Verification items for the finished model (mm, model axes). A direction names the side the tool comes from. Give positions to 0.01 mm unless a question says otherwise; leave off trailing zeros. Loops run counter-clockwise (first coordinate to the right, second up) from the corner with the lowest first, then second, coordinate; pieces in that order, holes last. Notation, with made-up numbers: (47.5, 35) - (98.5, 35) arc R28 ccw to (98.5, 60) - close; hole circle Ø8 at (-2, -37.75). An arc over 180 degrees is marked (long way). Answer in a Markdown table with one row per item.
```python
from build123d import *

# Parameters (mm, degrees)
F1_DEPTH = 254


with BuildPart() as f1:
    # F0 (on Front) → F1 (new body)
    with BuildSketch(Plane.XZ):
        Polygon((124.411419, 0), (0, 0), (0, -63.5), (63.5, -63.5), (48.04277, -25.4), (201.770738, -25.4), (190.5, -63.5), (254, -63.5), (254, 0), align=None)
        with BuildLine():
            Line((37.633552, 108.208333), (0, 0))
            Line((0, 0), (124.411419, 0))
            ThreePointArc((124.411419, 0), (55.058262, 33.282111), (37.633552, 108.208333))
        make_face()
        with BuildLine():
            ThreePointArc((213.311419, 88.9), (187.273212, 26.038207), (124.411419, 0))
            Line((124.411419, 0), (254, 0))
            Line((254, 0), (211.189286, 108.208333))
            ThreePointArc((211.189286, 108.208333), (212.779293, 98.612301), (213.311419, 88.9))
        make_face()
    extrude(amount=F1_DEPTH)


solid = f1.part
```
Q1. Draft check along Z on faces 1 (the face through (212.764, -125.222, 98.748)), 2 (the face through (0, -125, -31)), 3 (the face through (222, -125, -63.5)). Enter one of: +Z half, -Z half, draft (parallel to the pull), parting line (faces both ways), or undercut.
Completed:
| item | result |
|---|---|
| face 1 | undercut |
| face 2 | draft |
| face 3 | -Z half |
Q2. Go/stop test with flat-tipped pins: P1, Ø3, axis at x = 86.5, y = -25.5, coming from the +Z side; P2, Ø1.5, axis at y = -225, z = 46, coming from the -X side; P3, Ø3, axis at x = 171.5, y = -197.5, coming from the -Z side. Record where each tip stops, or that it passes through.
Completed:
| item | result |
|---|---|
| P1 | z = 9.21 |
| P2 | x = 15.74 |
| P3 | z = -25.4 |
Q3. Thickness scan on line 1 (X direction, y = -228.5, z = 22); line 2 (X direction, y = -25, z = 35.5); line 3 (Z direction, x = 185, y = -144.5). Record the ranges inside material, lowest first.
Completed:
| item | result |
|---|---|
| line 1 | 7.65 to 65.87, 182.96 to 245.3 |
| line 2 | 12.35 to 53.34, 195.49 to 239.96 |
| line 3 | -25.4 to 23.84 |
Q4. Sectioned sample at A-A (y = -164). Record the cut outline in (x, z).
Completed:
| item | result |
|---|---|
| outline | (0, -63.5) - (63.5, -63.5) - (48.04, -25.4) - (201.77, -25.4) - (190.5, -63.5) - (254, -63.5) - (254, 0) - (211.19, 108.21) arc R88.9 cw to (213.31, 88.9) arc R88.9 cw (long way) to (37.63, 108.21) - (0, 0) - close |
Q5. Sectioned sample at D-D (x = 148). Record the cut outline in (y, z), and give its area (3 significant figures).
Completed:
| item | result |
|---|---|
| outline | (-254, -25.4) - (0, -25.4) - (0, 3.19) - (-254, 3.19) - close |
| area | 7,260 mm^2 |
Q6. Sectioned sample at C-C (z = 28.5). Record the cut outline in (x, y), and give its area (3 significant figures).
Completed:
| item | result |
|---|---|
| outline | (9.91, -254) - (59.18, -254) - (59.18, 0) - (9.91, 0) - close; (189.64, -254) - (242.72, -254) - (242.72, 0) - (189.64, 0) - close |
| area | 26,000 mm^2 |
Q7. Tool access check on faces 4 (the face through (125, -254, -15)), 5 (the face through (196.214, -125.222, -44.183)). Record the directions out of +Z, -Z, +X, -X, +Y, -Y that give a thin tool (end or side, any length) a straight path to the whole face; none if there is none.
Completed:
| item | result |
|---|---|
| face 4 | +Z, -Z, +X, -X, -Y |
| face 5 | +Y, -Y |
Q8. Sectioned sample at B-B (z = -53). Record the cut outline in (x, y).
Completed:
| item | result |
|---|---|
| outline | (0, -254) - (59.24, -254) - (59.24, 0) - (0, 0) - close; (193.61, -254) - (254, -254) - (254, 0) - (193.61, 0) - close |
